```python
from build123d import *

# Parameters (mm, degrees)
F1_DEPTH = 5.08
F2_R     = 5.08


with BuildPart() as f1:
    # F0 (on Top) → F1 (new body)
    with BuildSketch(Plane.XY):
        with BuildLine():
            Line((25.277688, 30.232569), (18.927688, 30.232569))
            Line((18.927688, 30.232569), (18.927688, -45.967431))
            Line((18.927688, -45.967431), (25.277688, -45.967431))
            Line((25.277688, -45.967431), (25.277688, -44.953016))
            ThreePointArc((25.277688, -44.953016), (23.903282, -43.57861), (25.277688, -42.204203))
            Line((25.277688, -42.204203), (25.277688, -39.617431))
            ThreePointArc((25.277688, -39.617431), (22.102688, -36.442431), (25.277688, -33.267431))
            Line((25.277688, -33.267431), (25.277688, -30.092431))
            ThreePointArc((25.277688, -30.092431), (22.102688, -26.917431), (25.277688, -23.742431))
            Line((25.277688, -23.742431), (25.277688, -20.567431))
            ThreePointArc((25.277688, -20.567431), (22.102688, -17.392431), (25.277688, -14.217431))
            Line((25.277688, -14.217431), (25.277688, -11.042431))
            ThreePointArc((25.277688, -11.042431), (22.102688, -7.867431), (25.277688, -4.692431))
            Line((25.277688, -4.692431), (25.277688, -1.517431))
            ThreePointArc((25.277688, -1.517431), (22.102688, 1.657569), (25.277688, 4.832569))
            Line((25.277688, 4.832569), (25.277688, 8.007569))
            ThreePointArc((25.277688, 8.007569), (22.102688, 11.182569), (25.277688, 14.357569))
            Line((25.277688, 14.357569), (25.277688, 17.532569))
            ThreePointArc((25.277688, 17.532569), (22.102688, 20.707569), (25.277688, 23.882569))
            Line((25.277688, 23.882569), (25.277688, 26.255571))
            ThreePointArc((25.277688, 26.255571), (24.325188, 27.208071), (25.277688, 28.160571))
            Line((25.277688, 28.160571), (25.277688, 30.232569))
        make_face()
        with BuildLine():
            Line((31.627688, 30.232569), (25.277688, 30.232569))
            Line((25.277688, 30.232569), (25.277688, 28.160571))
            ThreePointArc((25.277688, 28.160571), (25.951207, 27.88159), (26.230188, 27.208071))
            ThreePointArc((26.230188, 27.208071), (25.951207, 26.534552), (25.277688, 26.255571))
            Line((25.277688, 26.255571), (25.277688, 23.882569))
            ThreePointArc((25.277688, 23.882569), (27.522752, 22.952633), (28.452688, 20.707569))
            ThreePointArc((28.452688, 20.707569), (27.522752, 18.462505), (25.277688, 17.532569))
            Line((25.277688, 17.532569), (25.277688, 14.357569))
            ThreePointArc((25.277688, 14.357569), (27.522752, 13.427633), (28.452688, 11.182569))
            ThreePointArc((28.452688, 11.182569), (27.522752, 8.937505), (25.277688, 8.007569))
            Line((25.277688, 8.007569), (25.277688, 4.832569))
            ThreePointArc((25.277688, 4.832569), (27.522752, 3.902633), (28.452688, 1.657569))
            ThreePointArc((28.452688, 1.657569), (27.522752, -0.587495), (25.277688, -1.517431))
            Line((25.277688, -1.517431), (25.277688, -4.692431))
            ThreePointArc((25.277688, -4.692431), (27.522752, -5.622367), (28.452688, -7.867431))
            ThreePointArc((28.452688, -7.867431), (27.522752, -10.112495), (25.277688, -11.042431))
            Line((25.277688, -11.042431), (25.277688, -14.217431))
            ThreePointArc((25.277688, -14.217431), (27.522752, -15.147367), (28.452688, -17.392431))
            ThreePointArc((28.452688, -17.392431), (27.522752, -19.637495), (25.277688, -20.567431))
            Line((25.277688, -20.567431), (25.277688, -23.742431))
            ThreePointArc((25.277688, -23.742431), (27.522752, -24.672367), (28.452688, -26.917431))
            ThreePointArc((28.452688, -26.917431), (27.522752, -29.162495), (25.277688, -30.092431))
            Line((25.277688, -30.092431), (25.277688, -33.267431))
            ThreePointArc((25.277688, -33.267431), (27.522752, -34.197367), (28.452688, -36.442431))
            ThreePointArc((28.452688, -36.442431), (27.522752, -38.687495), (25.277688, -39.617431))
            Line((25.277688, -39.617431), (25.277688, -42.204203))
            ThreePointArc((25.277688, -42.204203), (26.24954, -42.606758), (26.652095, -43.57861))
            ThreePointArc((26.652095, -43.57861), (26.24954, -44.550462), (25.277688, -44.953016))
            Line((25.277688, -44.953016), (25.277688, -45.967431))
            Line((25.277688, -45.967431), (31.627688, -45.967431))
            Line((31.627688, -45.967431), (31.627688, 30.232569))
        make_face()
    extrude(amount=F1_DEPTH)

    # F2
    f2_edges = [f1.edges().sort_by_distance(p)[0] for p in [
        (31.627688, 30.232569, 2.54),
        (18.927688, 30.232569, 2.54),
    ]]
    fillet(f2_edges, radius=F2_R)


solid = f1.part
```
Geometry: final body of the model. Coordinates: model frame, mm. Coordinates: 2 decimals unless noted, no trailing zeros. Order: outer loops, then holes, each group sorted by start corner. A loop starts at its lowest first (then second) coordinate and runs counter-clockwise, first axis right, second up. Notation, with made-up numbers: (57, -25) -> (104, -25) arc R16 cw to (104, 6) -> close; hole circle Ø11 at (33, -7.75). An arc over 180 degrees is marked (long way). Answer in a Markdown table with one row per item.
Item 1: Section B-B on y = -6. Output: boundary loops of the cut face in (x, z), plus the area to 3 significant figures.
Return value:
| item | result |
|---|---|
| outline | (18.93, 0) -> (22.71, 0) -> (22.71, 5.08) -> (18.93, 5.08) -> close; (27.85, 0) -> (31.63, 0) -> (31.63, 5.08) -> (27.85, 5.08) -> close |
| area | 38.4 mm² |
Item 2: Ray query, L1, parallel to X at y = -8, z = 0.4; L2, parallel to X at y = 20, z = 1.45; L3, parallel to Y at x = 19.5, z = 4. Return the intervals inside material, ascending.
Return value:
| item | result |
|---|---|
| L1 | x = 18.93 to 22.11, 28.45 to 31.63 |
| L2 | x = 18.93 to 22.18, 28.37 to 31.63 |
| L3 | y = -45.97 to 27.5 |
Item 3: Section D-D on y = 10. Output: boundary loops of the cut face in (x, z).
Return value:
| item | result |
|---|---|
| outline | (18.93, 0) -> (22.33, 0) -> (22.33, 5.08) -> (18.93, 5.08) -> close; (28.22, 0) -> (31.63, 0) -> (31.63, 5.08) -> (28.22, 5.08) -> close |
Item 4: Contact query for a flat-ended pin moving along its axis: P1, Ø2, axis at x = 23.5, z = 1, coming from the +Y side. Output: stop coordinate, or through.
Return value:
| item | result |
|---|---|
| P1 | stops at y = 30.23 |
Item 5: Section A-A on z = 3.9. State how many separate pieces and enclosed holes the cut face has, plus the area to 3 significant figures.
Return value:
| item | result |
|---|---|
| separate pieces | 1 |
| enclosed holes | 9 |
| area | 726 mm² |
